```python
from build123d import *

# Parameters (mm, degrees)
SKETCH_1_R               = 13.5
SKETCH_1_R_2             = 1.5
EXTRUDE_1_DEPTH          = 2
SKETCH_2_R               = 7
EXTRUDE_2_DEPTH          = 5
CUT_EXTRUDE_1_DEPTH      = 21.334699408
CUT_EXTRUDE_2_DEPTH      = 24.184046239
CUT_EXTRUDE_2_DEPTH_BACK = 24.184046239
SKETCH_4_R               = 1.5
CUT_EXTRUDE_START        = -2
SKETCH_5_R               = 5
CUT_EXTRUDE_3_DEPTH      = 2


with BuildPart() as part:
    # 草图1 → 凸台-拉伸1 (new body)
    with BuildSketch(Plane.XY):
        Circle(SKETCH_1_R)
        with Locations((6.717514421, 6.717514421)):
            Circle(SKETCH_1_R_2, mode=Mode.SUBTRACT)
        with Locations((6.717514421, -6.717514421)):
            Circle(SKETCH_1_R_2, mode=Mode.SUBTRACT)
        with Locations((-6.717514421, -6.717514421)):
            Circle(SKETCH_1_R_2, mode=Mode.SUBTRACT)
        with Locations((-6.717514421, 6.717514421)):
            Circle(SKETCH_1_R_2, mode=Mode.SUBTRACT)
    extrude(amount=EXTRUDE_1_DEPTH)

    # 草图2 → 凸台-拉伸2 (add)
    with BuildSketch(Plane.XY.offset(2)):
        Circle(SKETCH_2_R)
    extrude(amount=EXTRUDE_2_DEPTH)

    # 草图3 → 切除-拉伸1 (cut, through all)
    with BuildSketch(Plane.XY.offset(7)):
        with BuildLine():
            Line((-3, 4), (3, 4))
            ThreePointArc((3, 4), (5, 0), (3, -4))
            Line((3, -4), (-3, -4))
            ThreePointArc((-3, -4), (-5, 0), (-3, 4))
        make_face()
    extrude(amount=-CUT_EXTRUDE_1_DEPTH, mode=Mode.SUBTRACT)

    # 草图4 → 切除-拉伸2 (cut, two sides: drawn at the far end of the back side and taken through both)
    with BuildSketch(Plane.XZ.offset(-4).offset(-CUT_EXTRUDE_2_DEPTH_BACK)):
        with Locations(Location((0, 4.5, 0), (0, 0, 270))):
            Circle(SKETCH_4_R)
    extrude(amount=CUT_EXTRUDE_2_DEPTH + CUT_EXTRUDE_2_DEPTH_BACK, mode=Mode.SUBTRACT)

    # 草图5 → 切除-拉伸3 (cut)
    with BuildSketch(Plane(origin=(0, 0, 0), x_dir=(-1, 0, 0), z_dir=(0, 0, -1)).offset(CUT_EXTRUDE_START)):
        with Locations(Location((0, 0, 0), (0, 0, 180))):
            Circle(SKETCH_5_R)
    extrude(amount=CUT_EXTRUDE_3_DEPTH, mode=Mode.SUBTRACT)


solid = part.part
```
Work out the finished part from the listing and answer in its coordinate system (mm). A direction names the side the tool comes from. Round coordinates to 2 decimals unless told otherwise and drop trailing zeros. Order: outer loops, then holes, each group sorted by start corner. A loop starts at its lowest first (then second) coordinate and runs counter-clockwise, first axis right, second up.
Q1. A tool of negligible diameter and unlimited length cuts with its end or side. For faces 4 (the flat face through (0, -4, 6.2)), 5 (the cylindrical face through (3.25, 3.8, 3.55)), 6 (the flat face through (9, 0, 2)), 7 (the flat face through (0, -5, 7)), 8 (the cylindrical face through (-0.575, 5.523, 3.114)), from which of +Z, -Z, +X, -X, +Y, -Y can it reach the whole face along a straight path? Write none if from no direction.
Solution:
face 4: +Z, -Z
face 5: -Z
face 6: +Z
face 7: +Z, +X, -X, +Y, -Y
face 8: +Y, -Y
Q2. A cutting plane is placed at A-A, the plane y = 0. Determine the outline of the cut face in (x, z).
Solution:
outline: (-13.5, 0) - (-5, 0) - (-5, 7) - (-7, 7) - (-7, 2) - (-13.5, 2) - close; (5, 0) - (13.5, 0) - (13.5, 2) - (7, 2) - (7, 7) - (5, 7) - close
Q3. A cutting plane is placed at D-D, the plane z = 4.75. Determine the outline of the cut face in (x, y).
Solution:
outline: (-3, -4) arc R5 cw to (-3, 4) - (-1.48, 4) - (-1.48, 6.84) arc R7 ccw to (-1.48, -6.84) - (-1.48, -4) - close; (1.48, -6.84) arc R7 ccw to (1.48, 6.84) - (1.48, 4) - (3, 4) arc R5 cw to (3, -4) - (1.48, -4) - close
Q4. The mould has two halves that part along X. Classify faces 1 (the cylindrical face through (3.23, -6.21, 4.46)), 2 (the cylindrical face through (0, -5, 6)), 3 (the flat face through (6, 0, 0)): pulls with the +X half, pulls with the -X half, needs draft (parallel to the pull), parting line crosses it, or undercut.
Solution:
face 1: parting line crosses it
face 2: undercut
face 3: needs draft
Q5. Find the intervals of material crossed by line 1 along X through (y, z) = (5.5, 1.5); line 2 along Z through (x, y) = (0, -5.5); line 3 along Z through (x, y) = (-7, -4.5), in increasing order.
Solution:
line 1: x = -12.33 to -7.59, -5.84 to 5.84, 7.59 to 12.33
line 2: z = 0 to 3, 6 to 7
line 3: z = 0 to 2
Q6. A cutting plane is placed at B-B, the plane x = 0. Determine the outline of the cut face in (y, z).
Solution:
outline: (-13.5, 0) - (-5, 0) - (-5, 2) - (-4, 2) - (-4, 3) - (-7, 3) - (-7, 2) - (-13.5, 2) - close; (-7, 6) - (-4, 6) - (-4, 7) - (-7, 7) - close; (4, 2) - (5, 2) - (5, 0) - (13.5, 0) - (13.5, 2) - (7, 2) - (7, 3) - (4, 3) - close; (4, 6) - (7, 6) - (7, 7) - (4, 7) - close
Q7. Given pin 1 Ø3.5 at (x, y) = (-6.72, -6.72) entering from +Z; pin 2 Ø1.5 at (x, z) = (6, 6) entering from +Y; pin 3 Ø0.8 at (x, y) = (0, -4.5) entering from -Z, each flat-ended and moving along its own axis, determine where each tip first touches the part or whether it passes through.
Solution:
pin 1: stops at z = 2
pin 2: stops at y = 4.63
pin 3: stops at z = 2
Q8. A cutting plane is placed at C-C, the plane y = -5.75. Determine the outline of the cut face in (x, z), then the cut area to 3 significant figures.
Solution:
outline: (-12.21, 0) - (-7.86, 0) - (-7.86, 2) - (-12.21, 2) - close; (-5.57, 0) - (5.57, 0) - (5.57, 2) - (3.99, 2) - (3.99, 7) - (-3.99, 7) - (-3.99, 2) - (-5.57, 2) - close; (7.86, 0) - (12.21, 0) - (12.21, 2) - (7.86, 2) - close; hole circle Ø3 at (0, 4.5)
area: 72.5 mm2
